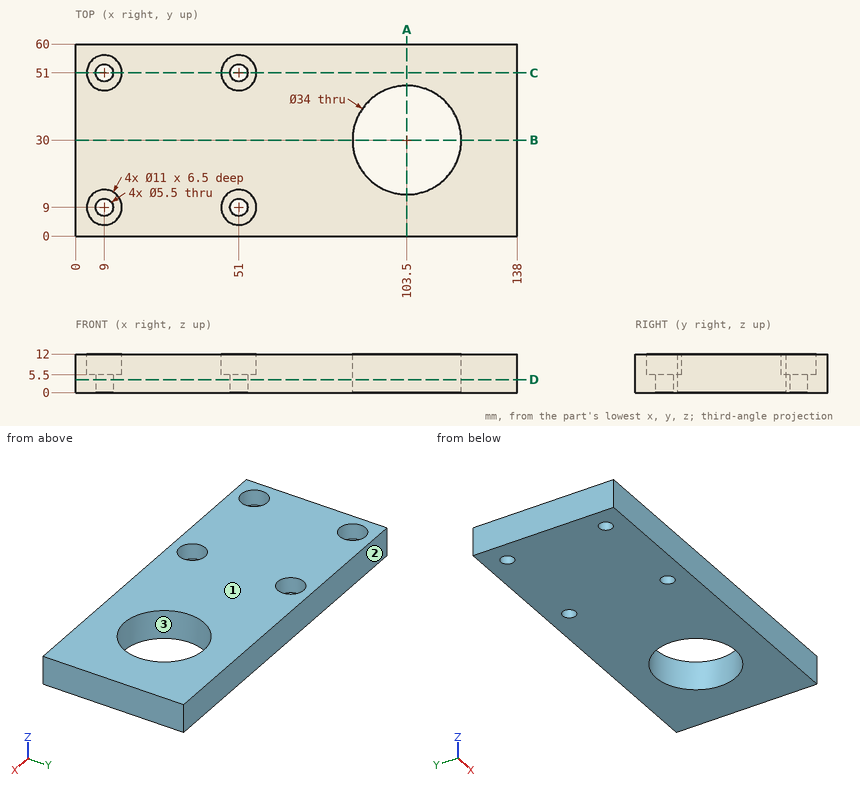
Could you check a few things on this drawing? It's one solid part, dimensions in mm from its lowest x, y, z. Coordinates: 2 decimals unless noted, no trailing zeros. Write each loop counter-clockwise with the first axis right and the second up, starting at its lowest first coordinate (ties: lowest second). Pieces come first, ordered by that corner, then holes. Notation, with made-up numbers: (80.25, -33) - (137.25, -33) arc R25 cw to (137.25, -5) - close; hole circle Ø11 at (51, -26.5). An arc over 180 degrees is marked (long way). Write item = value, one per line.
1) Suppose I cut it at B-B on y = 30. Please give me the cut outline in (x, z).
Result set:
outline = (0, 0) - (86.5, 0) - (86.5, 12) - (0, 12) - close; (120.5, 0) - (138, 0) - (138, 12) - (120.5, 12) - close
2) Will this pin go through, and if not, where does the flat tip stop? pin 1 Ø9 at (x, y) = (51, 51) entering from +Z.
Result set:
pin_1 = 5.5
3) Suppose I cut it at D-D on z = 4. Please give me the cut outline in (x, y).
Result set:
outline = (0, 0) - (138, 0) - (138, 60) - (0, 60) - close; hole circle Ø5.5 at (9, 9); hole circle Ø5.5 at (9, 51); hole circle Ø5.5 at (51, 9); hole circle Ø5.5 at (51, 51); hole circle Ø34 at (103.5, 30)
4) Please list where these lines run through material, in increasing order: line 1 (Y direction, x = 51, z = 1.6); line 2 (X direction, y = 51, z = 9.25); line 3 (X direction, y = 51, z = 3.4). Write a range as [from, to].
Result set:
line_1 = [0, 6.25], [11.75, 48.25], [53.75, 60]
line_2 = [0, 3.5], [14.5, 45.5], [56.5, 138]
line_3 = [0, 6.25], [11.75, 48.25], [53.75, 138]
5) We'd pull the mould along Y, two halves only. Please class the marked faces 1, 2 and 3: +Y half, -Y half, draft (parallel to the pull), parting line (faces both ways), or undercut.
Result set:
face_1 = draft
face_2 = +Y half
face_3 = undercut
6) Suppose I cut it at A-A on x = 103.5. Please give me the cut outline in (y, z).
Result set:
outline = (0, 0) - (13, 0) - (13, 12) - (0, 12) - close; (47, 0) - (60, 0) - (60, 12) - (47, 12) - close
7) Suppose I cut it at C-C on y = 51. Please give me the cut outline in (x, z), plus the area to 3 significant figures.
Result set:
outline = (0, 0) - (6.25, 0) - (6.25, 5.5) - (3.5, 5.5) - (3.5, 12) - (0, 12) - close; (11.75, 0) - (48.25, 0) - (48.25, 5.5) - (45.5, 5.5) - (45.5, 12) - (14.5, 12) - (14.5, 5.5) - (11.75, 5.5) - close; (53.75, 0) - (138, 0) - (138, 12) - (56.5, 12) - (56.5, 5.5) - (53.75, 5.5) - close
area = 1,450 mm2
